The model under review builds one solid part; all positions refer to its coordinate system, in mm. A direction names the side the tool comes from. Coordinates: 2 decimals unless noted, no trailing zeros. Write each loop counter-clockwise with the first axis right and the second up, starting at its lowest first coordinate (ties: lowest second). Pieces come first, ordered by that corner, then holes. Notation, with made-up numbers: (14, 27.5) -> (40, 27.5) arc R13 ccw to (40, 46.5) -> close; hole circle Ø7 at (71, 48.25). An arc over 180 degrees is marked (long way). Write each question's results on one line, items separated by ' | '.
```python
from build123d import *

# Parameters (mm, degrees)
CROQUIS1_W              = 100
CROQUIS1_H              = 100
SALIENTE_EXTRUIR1_DEPTH = 150
SALIENTE_EXTRUIR2_DEPTH = 100
VACIADO4_T              = -10


with BuildPart() as part:
    # Croquis1 → Saliente-Extruir1 (new body)
    with BuildSketch(Plane(origin=(0, 0, 0), x_dir=(1, 0, 0), z_dir=(0, 1, 0))):
        with Locations((50, 50)):
            Rectangle(CROQUIS1_W, CROQUIS1_H)
    extrude(amount=SALIENTE_EXTRUIR1_DEPTH)

    # Croquis2 → Saliente-Extruir2 (add)
    with BuildSketch(Plane.XY):
        Polygon((0, 0), (0, -57.735026919), (100, 0), align=None)
    extrude(amount=-SALIENTE_EXTRUIR2_DEPTH)

    # Vaciado4
    vaciado4_openings = [part.faces().sort_by_distance(p)[0] for p in [
        (50, 150, -50),
    ]]
    offset(amount=VACIADO4_T, openings=vaciado4_openings, kind=Kind.INTERSECTION)


solid = part.part
```
Q1. Machinability: for faces 1 (the flat face through (100, 74, -49)), 2 (the flat face through (49, 56, -10)), which of the approach directions +Z, -Z, +X, -X, +Y, -Y give a long, thin tool a straight path to every point of the face, cutting with its end or side? Answer none if there is none.
Solution:
face 1: +Z, -Z, +X, +Y, -Y | face 2: +Y
Q2. Add section B-B (z = -49). Write out the cut boundary in (x, y).
Solution:
outline: (0, -57.74) -> (100, 0) -> (100, 150) -> (90, 150) -> (90, 5.77) -> (10, -40.41) -> (10, 150) -> (0, 150) -> close
Q3. Clearance check with flat-ended pins moving along their axes: P1, Ø3, axis at y = -5.5, z = -87, coming from the +X side; P2, Ø6, axis at x = 51.5, z = -19.5, coming from the -Y side; P3, Ø10, axis at x = 64, z = -49, coming from the +Y side. State where each tip first meets the part, or that it passes through.
Solution:
P1: x = 93.07 | P2: y = -29.73 | P3: y = -6.35
Q4. For line 1 (Z direction, x = 64, y = 39); line 2 (X direction, y = 51, z = -50); line 3 (X direction, y = -31, z = -67), list the stretches that pass through material, from the lowest coordinate up. Write a range as from..to.
Solution:
line 1: -100..-90, -10..0 | line 2: 0..10, 90..100 | line 3: 0..10, 26.31..46.31
Q5. Add section D-D (y = -12). Write out the cut boundary in (x, z).
Solution:
outline: (0, -100) -> (79.22, -100) -> (79.22, 0) -> (0, 0) -> close; hole (10, -90) -> (59.22, -90) -> (59.22, -10) -> (10, -10) -> close
Q6. Draft analysis for pull direction X (two halves, no side actions). For faces 3 (the flat face through (49, 71, 0)), 4 (the flat face through (49.3, -29.27, -49.3)), 5 (the flat face through (49.44, -17.644, -49.44)), state which applies: pulls with the +X half, pulls with the -X half, needs draft (parallel to the pull), parting line crosses it, or undercut.
Solution:
face 3: needs draft | face 4: pulls with the +X half | face 5: undercut
Q7. Add section A-A (y = 26). Write out the cut boundary in (x, z).
Solution:
outline: (0, -100) -> (100, -100) -> (100, 0) -> (0, 0) -> close; hole (10, -90) -> (90, -90) -> (90, -10) -> (10, -10) -> close
Q8. Add section C-C (x = 84.5). Write out the cut boundary in (y, z).
Solution:
outline: (-8.95, -100) -> (150, -100) -> (150, -90) -> (2.6, -90) -> (2.6, -10) -> (150, -10) -> (150, 0) -> (-8.95, 0) -> close
